from build123d import *

# Parameters (mm, degrees)
F1_DEPTH = 2
F3_DEPTH = 10


# Not quite as in the source:
# - a feature names something its author has since deleted; it is built from what else it names


with BuildPart() as f1:
    # F0 (on Top) → F1 (new body)
    with BuildSketch(Plane.XY):
        Polygon((-5.0628672683, -46.2001158912), (37.4790403854, -27.4846296159), (42.5419076537, 18.7154862752), (5.0628672683, 46.2001158912), (-37.4790403854, 27.4846296159), (-42.5419076537, -18.7154862752), align=None)
        Polygon((-38.3141404334, -16.8555621733), (-33.7544152539, 24.7532378529), (4.5597251795, 41.6088000262), (38.3141404334, 16.8555621733), (33.7544152539, -24.7532378529), (-4.5597251795, -41.6088000262), align=None, mode=Mode.SUBTRACT)
    extrude(amount=F1_DEPTH)

    # F2 (on face) → F3 (join)
    with BuildSketch(Plane.XY.offset(2)):
        Polygon((-15.5215827184, 37.1443867888), (-16.8945903987, 36.5403587183), (-16.0086825619, 34.5266141206), (-17.3816902422, 33.9225860501), (-16.7776621717, 32.5495783698), (-12.6586391309, 34.3616625813), (-13.2626672014, 35.7346702616), (-14.6356748817, 35.1306421911), align=None)
        Polygon((24.4071912079, 32.0142783355), (23.1975837141, 32.9013238309), (21.8965836541, 31.12723284), (20.6869761604, 32.0142783355), (19.7999306649, 30.8046708417), (23.4287531463, 28.1435343554), (24.3157986417, 29.3531418491), (23.1061911479, 30.2401873446), align=None)
        Polygon((37.7418660296, -4.8904548465), (39.9287739263, -5.1301084533), (40.0921741128, -3.6390348874), (37.905266216, -3.3993812806), (38.0686664025, -1.9083077146), (36.5775928366, -1.7449075281), (36.0873922772, -6.218128226), (37.5784658431, -6.3815284124), align=None)
        Polygon((14.6356748817, -35.1306421911), (15.5215827184, -37.1443867888), (16.8945903987, -36.5403587183), (16.0086825619, -34.5266141206), (17.3816902422, -33.9225860501), (16.7776621717, -32.5495783698), (12.6586391309, -34.3616625813), (13.2626672014, -35.7346702616), align=None)
        Polygon((-23.1061911479, -30.2401873446), (-24.4071912079, -32.0142783355), (-23.1975837141, -32.9013238309), (-21.8965836541, -31.12723284), (-20.6869761604, -32.0142783355), (-19.7999306649, -30.8046708417), (-23.4287531463, -28.1435343554), (-24.3157986417, -29.3531418491), align=None)
        Polygon((-39.9287739263, 5.1301084533), (-40.0921741128, 3.6390348874), (-37.905266216, 3.3993812806), (-38.0686664025, 1.9083077146), (-36.5775928366, 1.7449075281), (-36.0873922772, 6.218128226), (-37.5784658431, 6.3815284124), (-37.7418660296, 4.8904548465), align=None)
    extrude(amount=F3_DEPTH)


solid = f1.part
Model file for the job. Use its own axes, mm. A direction names the side the tool comes from. Coordinates: 2 decimals unless noted, no trailing zeros. Write each loop counter-clockwise with the first axis right and the second up, starting at its lowest first coordinate (ties: lowest second). Pieces come first, ordered by that corner, then holes. Notation, with made-up numbers: (4, 11) -> (56, 11) arc R20 cw to (56, 33) -> close; hole circle Ø9 at (13.5, 30.5). An arc over 180 degrees is marked (long way). One line per item, written item: value. Start each with the question number.
1) Slice it at C-C on x = 26. Write the cut outline in (y, z), then the cut area to 3 significant figures.
2) Flat gauge pins, fed straight in: pin 1 Ø6 at (x, z) = (27, 5.5) entering from -Y; pin 2 Ø10 at (x, y) = (-26.5, 30.5) entering from +Z; pin 3 Ø6 at (y, z) = (-8.5, 3) entering from +X; pin 4 Ø5 at (x, z) = (7, 1.5) entering from +Y. Where does each tip first touch, or does it go through?
3) Probe probe 1 along X at (y, z) = (-35.5, 7.5); probe 2 along X at (y, z) = (35.5, 4.25); probe 3 along Z at (x, y) = (36.5, -26). List the from-to ranges inside material, lowest first.
4) Which spindle directions (+Z, -Z, +X, -X, +Y, -Y) get a long thin tool onto all of the face, cutting with end or side? Do faces 4 (the face through (16.46, -35.55, 6.93)), 5 (the face through (38.82, -5.01, 6.93)), 6 (the face through (-36.336, 3.95, 6.93)). Say none if no direction does.
5) Slice it at A-A on x = 3.5. Write the cut outline in (y, z), then the cut area to 3 significant figures.
6) Pull direction X, two halves, no side cores. Call faces 1 (the face through (-39.01, 3.52, 6.93)), 2 (the face through (21.201, 29.405, 0.986)), 3 (the face through (23, 31, 12)): +X half, -X half, draft (parallel to the pull), parting line (faces both ways), or undercut.
7) Slice it at B-B on z = 8.5. Count the separate pieces of the cut face and the enclosed holes in it, then the cut area to 3 significant figures.
Answers follow:
1. outline: (-32.53, 0) -> (-28.16, 0) -> (-28.16, 2) -> (-32.53, 2) -> close; (25.89, 0) -> (30.85, 0) -> (30.85, 2) -> (25.89, 2) -> close
1. area: 18.7 mm2
2. pin 1: y = 28.92
2. pin 2: z = 2
2. pin 3: x = 39.87
2. pin 4: y = 46.2
3. probe 1: 13.16 to 13.8, 14.8 to 16.44
3. probe 2: -16.44 to -14.8, -13.8 to -13.16
3. probe 3: 0 to 2
4. face 4: +Z, +X
4. face 5: +Z, -Y
4. face 6: +Z, +X, -Y
5. outline: (-42.43, 0) -> (-38.06, 0) -> (-38.06, 2) -> (-42.43, 2) -> close; (41.14, 0) -> (45.51, 0) -> (45.51, 2) -> (41.14, 2) -> close
5. area: 17.5 mm2
6. face 1: -X half
6. face 2: undercut
6. face 3: draft
7. separate pieces: 6
7. enclosed holes: 0
7. area: 60.3 mm2
